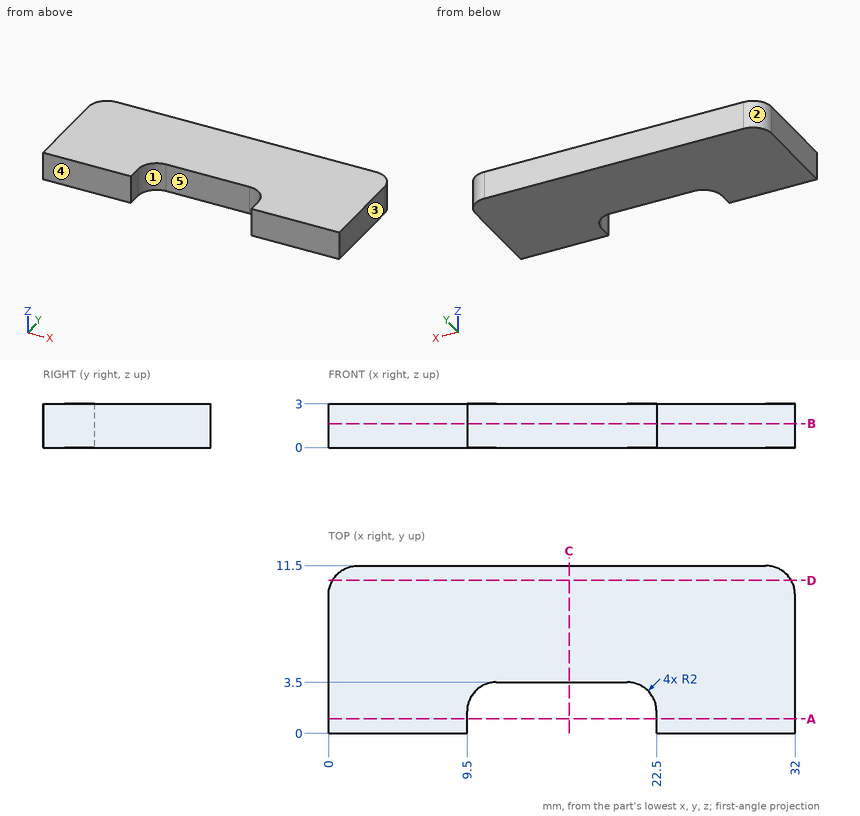
Answer from the drawing. Dimensions are ordinates in mm from the lowest x, y and z of the part. A direction names the side the tool comes from. Coordinates: 2 decimals unless noted, no trailing zeros. Order: outer loops, then holes, each group sorted by start corner. A loop starts at its lowest first (then second) coordinate and runs counter-clockwise, first axis right, second up. Notation, with made-up numbers: (78.5, -29.5) - (103.5, -29.5) arc R15 ccw to (103.5, -0.5) - close; hole circle Ø6 at (7.25, 68.25). An arc over 180 degrees is marked (long way). Answer as a JSON object with one key per item and string values. Group by question number.
Item 1: Section A-A (y = 1) is taken. Give the vertices of the cut face in (x, z), plus the area to 3 significant figures.
Item 2: The mould has two halves that part along X. Classify the marked faces 1, 2 and 3: +X half, -X half, draft (parallel to the pull), parting line (faces both ways), or undercut.
Item 3: A tool of negligible diameter and unlimited length cuts with its end or side. For the marked faces 4 and 5, from which of +Z, -Z, +X, -X, +Y, -Y can it reach the whole face along a straight path? Write none if from no direction.
Item 4: Section B-B (z = 1.65) is taken. Give the vertices of the cut face in (x, y).
Item 5: Section C-C (x = 16.5) is taken. Give the vertices of the cut face in (y, z).
Item 6: Flat-ended cylindrical pins translate along their axes: P1, Ø0.8, axis at y = 0.5, z = 1.5, coming from the -X side; P2, Ø1.5, axis at x = 20, z = 0.5, coming from the -Y side. Find the tip coordinate at first contact, or state that the pin passes through.
Item 7: Section D-D (y = 10.5) is taken. Give the vertices of the cut face in (x, z).
Item 8: Consider probe 1 along X at (y, z) = (0.75, 2); probe 2 along X at (y, z) = (2.5, 2.05); probe 3 along Y at (x, z) = (20, 0.2). Determine where each line is inside the solid, lowest interval first. Write a range as from..to.
Results are:
{
 "1": {"outline": "(0, 0) - (9.5, 0) - (9.5, 3) - (0, 3) - close; (22.5, 0) - (32, 0) - (32, 3) - (22.5, 3) - close", "area": "57.0 mm^2"},
 "2": {"face 1": "undercut", "face 2": "-X half", "face 3": "+X half"},
 "3": {"face 4": "+Z, -Z, +X, -X, -Y", "face 5": "+Z, -Z, -Y"},
 "4": {"outline": "(0, 0) - (9.5, 0) - (9.5, 1.5) arc R2 cw to (11.5, 3.5) - (20.5, 3.5) arc R2 cw to (22.5, 1.5) - (22.5, 0) - (32, 0) - (32, 9.5) arc R2 ccw to (30, 11.5) - (2, 11.5) arc R2 ccw to (0, 9.5) - close"},
 "5": {"outline": "(3.5, 0) - (11.5, 0) - (11.5, 3) - (3.5, 3) - close"},
 "6": {"P1": "stops at x = 0", "P2": "stops at y = 3.48"},
 "7": {"outline": "(0.27, 0) - (31.73, 0) - (31.73, 3) - (0.27, 3) - close"},
 "8": {"probe 1": "x = 0..9.5, 22.5..32", "probe 2": "x = 0..9.77, 22.23..32", "probe 3": "y = 3.5..11.5"}
}
